Design review of the part built by this model. Coordinates are the model's own, in mm. Face numbers are marked on the shaded views. A direction names the side the tool comes from. Give positions to 0.01 mm unless a question says otherwise; leave off trailing zeros. Loops run counter-clockwise (first coordinate to the right, second up) from the corner with the lowest first, then second, coordinate; pieces in that order, holes last. Notation, with made-up numbers: M 32,-35 L 52,-35 A14 ccw 52,-10 Z; hole C -35.5,82.25 d5. An arc over 180 degrees is marked long. Use a Markdown table: item, result. Add a question column.
(1) Insertion check: pin 1 Ø1.4 at (y, z) = (30, 2.5) entering from +X; pin 2 Ø6 at (y, z) = (36, 16.5) entering from +X; pin 3 Ø2 at (y, z) = (10, 2.5) entering from +X (3 decimals). Each pin has a flat end and moves straight along its axis. Give the tip position at first contact, or say it passes through.
(2) Add section A-A, the plane y = 20. Give the boundary of the cut face in (x, z).
(3) Add section C-C, the plane x = 12. Give the boundary of the cut face in (y, z).
(4) Add section D-D, the plane z = 23. Give the boundary of the cut face in (x, y), then the cut area to 3 significant figures.
(5) Draft analysis for pull direction Y (two halves, no side actions). For the marked faces 3, 4 and 5, state which applies: pulls with the +Y half, pulls with the -Y half, needs draft (parallel to the pull), parting line crosses it, or undercut.
(6) For probe 1 along Z at (x, y) = (30.55, 30); probe 2 along Y at (x, z) = (30.15, 47.5); probe 3 along Z at (x, y) = (7.5, 17), list the stretches that pass through material, from the lowest coordinate up.
(7) Add section B-B, the plane x = 31.5. Give the boundary of the cut face in (y, z), then the cut area to 3 significant figures.
(8) For the marked faces 1 and 2, list the 3-axis set-ups (+Z, -Z, +X, -X, +Y, -Y) from which the entire face can be reached by the end or side of a thin tool; tool diameter is ignored.
```python
from build123d import *

# Parameters (mm, degrees)
BOSS_EXTRUDE1_DEPTH         = 40
CUT_EXTRUDE1_REACH          = 74.265
SKETCH2_R                   = 5
M2_TAPPED_HOLE2_D           = 1.6
M2_TAPPED_HOLE2_DEPTH       = 5
M2_TAPPED_HOLE2_CSINK_D     = 2.05
M2_TAPPED_HOLE2_CSINK_ANGLE = 90
M2_TAPPED_HOLE2_TIP         = 0.480688495


with BuildPart() as part:
    # Sketch1 → Boss-Extrude1 (new body)
    with BuildSketch(Plane(origin=(0, 0, 0), x_dir=(1, 0, 0), z_dir=(0, 1, 0))):
        Polygon((33.5, 0), (33.5, -5), (5, -5), (5, -45), (33.5, -45), (33.5, -50), (0, -50), (0, 0), align=None)
    extrude(amount=BOSS_EXTRUDE1_DEPTH)

    # Sketch2 → Cut-Extrude1 (cut, up to next)
    with BuildSketch(Plane.ZY, mode=Mode.PRIVATE) as cut_extrude1_sk1:
        with Locations((25, 20)):
            Circle(SKETCH2_R)
    cut_extrude1_tool1 = extrude(cut_extrude1_sk1.sketch, amount=-CUT_EXTRUDE1_REACH, mode=Mode.PRIVATE) & part.part
    add(cut_extrude1_tool1.solids().sort_by_distance((0, 20, 25))[0], mode=Mode.SUBTRACT)

    # M2 Tapped Hole2
    with Locations(Plane(origin=(33.5, 30, 47.5), x_dir=(0, 0, 1), z_dir=(1, 0, 0))):
        with Locations((0, 0), (0, 20), (-45, 20), (-45, 0)):
            CounterSinkHole(M2_TAPPED_HOLE2_D / 2, M2_TAPPED_HOLE2_CSINK_D / 2, depth=M2_TAPPED_HOLE2_DEPTH, counter_sink_angle=M2_TAPPED_HOLE2_CSINK_ANGLE)
            with Locations((0, 0, -(M2_TAPPED_HOLE2_DEPTH + M2_TAPPED_HOLE2_TIP / 2))):  # 118° drill point
                Cone(0, M2_TAPPED_HOLE2_D / 2, M2_TAPPED_HOLE2_TIP, mode=Mode.SUBTRACT)


solid = part.part
```
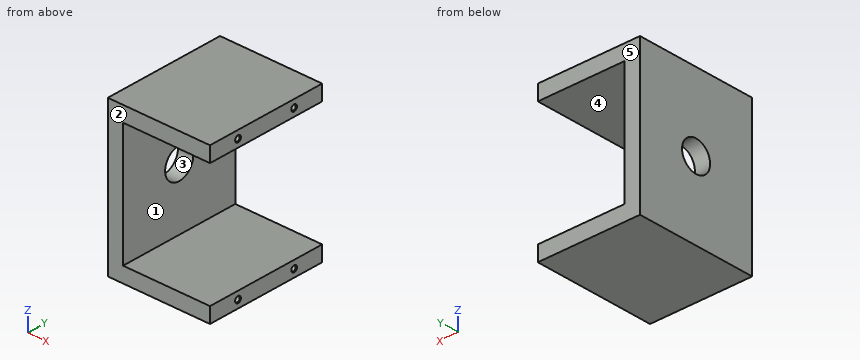
Established:
| question | item | result |
|---|---|---|
| 1 | pin 1 | x = 28.44 |
| 1 | pin 2 | x = 5 |
| 1 | pin 3 | x = 33.475 |
| 2 | outline | M 0,0 L 33.5,0 L 33.5,5 L 5,5 L 5,20 L 0,20 Z; M 0,30 L 5,30 L 5,45 L 33.5,45 L 33.5,50 L 0,50 Z |
| 3 | outline | M 0,0 L 40,0 L 40,5 L 0,5 Z; M 0,45 L 40,45 L 40,50 L 0,50 Z |
| 4 | outline | M 0,0 L 5,0 L 5,15.42 L 0,15.42 Z; M 0,24.58 L 5,24.58 L 5,40 L 0,40 Z |
| 4 | area | 154 mm^2 |
| 5 | face 3 | undercut |
| 5 | face 4 | needs draft |
| 5 | face 5 | pulls with the +Y half |
| 6 | probe 1 | 0 to 1.7, 3.3 to 5, 45 to 46.7, 48.3 to 50 |
| 6 | probe 2 | 0 to 9.2, 10.8 to 29.2, 30.8 to 40 |
| 6 | probe 3 | 0 to 5, 45 to 50 |
| 7 | outline | M 0,0 L 40,0 L 40,5 L 0,5 Z; M 0,45 L 40,45 L 40,50 L 0,50 Z; hole C 10,2.5 d1.6; hole C 10,47.5 d1.6; hole C 30,2.5 d1.6; hole C 30,47.5 d1.6 |
| 7 | area | 392 mm^2 |
| 8 | face 1 | +X, +Y, -Y |
| 8 | face 2 | +Z, -Z, +X, -X, -Y |
